Autodesk Inventor part; units mm, degrees
ref_plane "Work Plane1" through (0, 0, -15) normal (0, 0, 1) x (1, 0, 0)
ref_plane "YZ Plane" through (0, 0, 0) normal (1, 0, 0) x (0, 1, 0)
ref_plane "XZ Plane" through (0, 0, 0) normal (0, 1, 0) x (-1, 0, 0)
sketch "Sketch1" plane through (0, 0, 0) normal (0, 0, 1) x (1, 0, 0)
  line L0 (0, 0) -> (25, 0)
  line L1 (25, 0) -> (25, 40)
  line L2 (25, 40) -> (0, 40)
  line L3 (0, 40) -> (0, 0)
  dimension "d1" = 25
  dimension "d2" = 40
  dimension "d3" = 25
extrude "Extrusion1" add sketch "Sketch1" against normal blind 30
sketch "Sketch2" plane through (25, 0, 0) normal (1, 0, 0) x (0, 0, -1)
  line L0 (0, 0) -> (30, 0)
  circle A0 centre (15, 6.56) radius 2.46
extrude "Extrusion2" cut sketch "Sketch2" against normal blind 30
sketch "Sketch3" plane through (0, 0, 0) normal (-1, 0, 0) x (0, 0, 1)
  line L0 (0, 0) -> (-30, 0)
  line L1 (-25.05, 0) -> (-4.95, 0)
  line L2 (-4.95, 0) -> (-4.95, 33.12)
  line L3 (-4.95, 33.12) -> (-25.05, 33.12)
  line L4 (-25.05, 33.12) -> (-25.05, 0)
  dimension "d11" = 20.1
extrude "Extrusion3" cut sketch "Sketch3" against normal blind 20
sketch "Sketch4" plane through (0, 0, 0) normal (0, -1, 0) x (1, 0, 0)
  line L0 (20, -4.95) -> (20, -25.05)
  line L1 (20, -15) -> (25, -15)
  line L2 (25, 0) -> (25, -30)
  line L3 (20, -8.025) -> (25, -8.025)
  line L4 (25, -8.025) -> (25, -21.975)
  line L5 (25, -21.975) -> (20, -21.975)
  line L6 (20, -21.975) -> (20, -8.025)
  line L7 (20, -8.025) -> (25, -21.975) construction
  line L8 (25, -8.025) -> (20, -21.975) construction
  line L9 (25, -12.54) -> (25, -17.46)
  point P0 (0, 0)
  point P1 (22.5, -15)
  dimension "d14" = 13.95
extrude "Extrusion4" add sketch "Sketch4" along normal blind 15
sketch "Sketch5" plane through (20, 0, 0) normal (-1, 0, 0) x (0, 0, 1)
  circle A0 centre (-15, 6.56) radius 2.46
  circle A1 centre (-15, 6.56) radius 4.7025
  circle A2 centre (-15, 6.56) radius 2.46
  circle A3 centre (-15, 6.56) radius 2.46
  point P0 (0, 0)
  dimension "d17" = 9.405
extrude "Extrusion5" cut sketch "Sketch5" against normal blind 2.1
sketch "Sketch6" plane through (25, 0, 0) normal (1, 0, 0) x (0, 0, -1)
  circle A0 centre (15, 6.56) radius 4.7025
  line L0 (15, 6.56) -> (15, 23.56)
  circle A1 centre (15, 23.56) radius 2.46
  point P0 (0, 0)
  dimension "d20" = 17
  dimension "d21" = 4.92
extrude "Extrusion6" cut sketch "Sketch6" against normal blind 10 contours A1
sketch "Sketch7" plane through (20, 0, 0) normal (-1, 0, 0) x (0, 0, 1)
  circle A0 centre (-15, 23.56) radius 2.46
  circle A1 centre (-15, 23.56) radius 4.7025
  point P0 (0, 0)
  dimension "d24" = 9.405
extrude "Extrusion7" cut sketch "Sketch7" against normal blind 2.1
sketch "Sketch9" plane through (25, 0, 0) normal (1, 0, 0) x (0, 0, -1)
  circle A0 centre (15, 6.56) radius 2.46
  circle A1 centre (15, 6.56) radius 2.46
  circle A2 centre (15, 23.56) radius 2.46
  circle A3 centre (15, 23.56) radius 2.46
  line L0 (30, 40) -> (30, 0)
  line L1 (30, 0) -> (30, 40)
  line L2 (30, 40) -> (0, 40)
  line L3 (0, 40) -> (0, 0)
  line L4 (0, 0) -> (8.025, 0)
  line L5 (21.975, 0) -> (21.975, -15)
  line L6 (21.975, -15) -> (8.025, -15)
  line L7 (8.025, -15) -> (8.025, 0)
  line L8 (0, 0) -> (8.025, 0)
  line L9 (21.975, 0) -> (30, 0)
extrude "Extrusion8" add sketch "Sketch9" along normal blind 5
sketch "Sketch10" plane through (0, 40, 0) normal (0, 1, 0) x (1, 0, 0)
  line L0 (0, 30) -> (30, 30)
  line L1 (30, 0) -> (0, 0)
  line L2 (0, 30) -> (30, 30)
  line L3 (30, 30) -> (30, 0)
  line L4 (30, 0) -> (0, 0)
  line L5 (0, 0) -> (0, 30)
extrude "Extrusion9" add sketch "Sketch10" along normal blind 30
sketch "Sketch12" plane through (30, 0, 0) normal (1, 0, 0) x (0, 0, -1)
  circle A0 centre (15, 6.56) radius 2.46
  line L0 (15, 6.56) -> (15, 15.06)
  circle A1 centre (15, 15.06) radius 2.525
  point P0 (0, 0)
  dimension "d31" = 8.5
  dimension "d33" = 5.05
extrude "Extrusion10" cut sketch "Sketch12" against normal blind 30 contours A1
sketch "Sketch14" plane through (0, 0, 0) normal (0, 0, 1) x (1, 0, 0)
  line L0 (30, 70) -> (0, 70)
  line L1 (0, 70) -> (0, 85)
  line L2 (30, 100) -> (15, 115)
  line L3 (-12, 115) -> (15, 115)
  line L4 (30, 0) -> (30, 70)
  line L5 (30, 100) -> (30, 70)
  line L6 (-9.5, 113.5) -> (-12, 115)
  line L7 (-9.5, 101.5) -> (-12, 100)
  line L8 (-7, 107.5) -> (-9.5, 101.5)
  line L9 (-7, 107.5) -> (-9.5, 113.5)
  line L10 (0, 100) -> (0, 85)
  line L11 (0, 100) -> (-12, 100)
  point P0 (0, 0)
  dimension "d49" = 15
  dimension "d61" = 12
extrude "Extrusion12" add sketch "Sketch14" against normal blind 30
sketch "Sketch15" plane through (0, 0, -25.05) normal (-1, 0, 0) x (0, 0, 1)
  line L0 (0, 33.12) -> (20.1, 33.12)
  line L1 (20.1, 33.12) -> (20.1, 0)
  line L2 (0, 33.12) -> (20.1, 33.12)
  line L3 (20.1, 33.12) -> (20.1, 31.1)
  line L4 (20.1, 31.1) -> (0, 31.1)
  line L5 (0, 31.1) -> (0, 33.12)
  point P0 (25.05, 0)
  dimension "d57" = 2.02
extrude "Extrusion13" add sketch "Sketch15" against normal blind 20
sketch "Sketch19" plane through (0, 0, 0) normal (0, 0, 1) x (1, 0, 0)
  line L0 (0, 100) -> (0, 0)
  line L1 (0, 100) -> (-12, 100)
  line L2 (0, 100) -> (-12, 100)
  line L3 (-12, 100) -> (-9.5, 101.5)
  line L4 (-12, 100) -> (-9.5, 101.5)
  line L5 (-9.5, 101.5) -> (-7, 107.5)
  line L6 (-9.5, 101.5) -> (-7, 107.5)
  line L7 (-7, 107.5) -> (-9.5, 113.5)
  line L8 (-7, 107.5) -> (-9.5, 113.5)
  line L9 (-9.5, 113.5) -> (-12, 115)
  line L10 (-9.5, 113.5) -> (-12, 115)
  line L11 (-12, 115) -> (15, 115)
  line L12 (-12, 115) -> (15, 115)
  line L13 (15, 115) -> (30, 100)
  line L14 (15, 115) -> (30, 100)
  line L15 (30, 100) -> (30, 90)
  line L16 (30, 0) -> (30, 100)
  line L17 (30, 90) -> (0, 90)
  line L18 (0, 0) -> (0, 100)
  line L19 (0, 90) -> (0, 100)
  dimension "d62" = 10
  dimension "d63" = 30
extrude "Extrusion14" add sketch "Sketch19" along normal blind 30
ref_plane "Work Plane1" through (0, 0, -15) normal (0, 0, 1) x (1, 0, 0)
mirror "Mirror1" about plane through (0, 0, -15) normal (0, 0, 1) of "Extrusion14"
properties part number "rec_b_12mm_x_90mm"
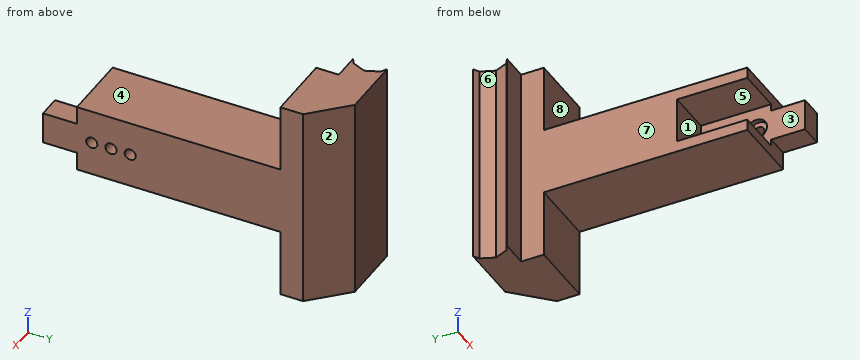
The model under review builds one solid part; all positions refer to its coordinate system, in mm. Face numbers are marked on the shaded views. A direction names the side the tool comes from. Round coordinates to 2 decimals unless told otherwise and drop trailing zeros. Loops run counter-clockwise (first coordinate to the right, second up) from the corner with the lowest first, then second, coordinate; pieces in that order, holes last. Notation, with made-up numbers: M -38.75,26 L 20.25,26 A29 ccw 20.25,53 Z; hole C 88.25,-35 d10. An arc over 180 degrees is marked long. Answer as a JSON object with one key per item and string values.
(1) To check wall thickness, follow line 1 along Z through (x, y) = (24.25, 6.56); line 2 along Y through (x, z) = (-9.5, -8); line 3 along Y through (x, z) = (26, -14). State the ranges of each line that lie inside material, in increasing order.
Resolved:
{"line 1": "-30 to -17.46, -12.54 to 0", "line 2": "100 to 101.5, 113.5 to 115", "line 3": "-15 to 4.31, 8.81 to 12.74, 17.38 to 21.31, 25.81 to 104"}
(2) Tool access review of the marked faces 5, 6, 7 and 8: name each direction out of +Z, -Z, +X, -X, +Y, -Y from which nothing blocks a thin tool from reaching the whole face with its end or side.
Resolved:
{"face 5": "-X, -Y", "face 6": "+Z, -Z, -X", "face 7": "+Z, -Z, -X, -Y", "face 8": "+Z, +X, -X, -Y"}
(3) Take a section at B-B on x = 7. Give the boundary of the cut face in (y, z).
Resolved:
{"outline": "M 0,-30 L 90,-30 L 90,-60 L 115,-60 L 115,30 L 90,30 L 90,0 L 0,0 L 0,-4.95 L 31.1,-4.95 L 31.1,-25.05 L 0,-25.05 Z"}
(4) Take a section at A-A on y = 6.56. Give the boundary of the cut face in (x, z), and give its area (3 significant figures).
Resolved:
{"outline": "M 0,-30 L 30,-30 L 30,-17.46 L 22.1,-17.46 L 22.1,-19.7 L 20,-19.7 L 20,-25.05 L 0,-25.05 Z; M 0,-4.95 L 20,-4.95 L 20,-10.3 L 22.1,-10.3 L 22.1,-12.54 L 30,-12.54 L 30,0 L 0,0 Z", "area": "439 mm²"}
(5) Take a section at D-D on x = 18.5. Give the boundary of the cut face in (y, z), and give its area (3 significant figures).
Resolved:
{"outline": "M 0,-30 L 90,-30 L 90,-60 L 111.5,-60 L 111.5,30 L 90,30 L 90,0 L 0,0 L 0,-4.95 L 31.1,-4.95 L 31.1,-25.05 L 0,-25.05 Z", "area": "4,010 mm²"}
(6) Clearance check with flat-ended pins moving along their axes: P1, Ø12, axis at y = 23.56, z = -15, coming from the +X side; P2, Ø6, axis at x = -5.5, z = -32, coming from the -Y side; P3, Ø9, axis at x = 8.5, z = -4.5, coming from the -Y side; P4, Ø5, axis at x = 27, y = -5, coming from the +Z side (3 decimals). State where each tip first meets the part, or that it passes through.
Resolved:
{"P1": "x = 30", "P2": "y = 100", "P3": "y = 0", "P4": "z = -8.025"}
(7) Draft analysis for pull direction Z (two halves, no side actions). For the marked faces 1, 2, 3 and 4, state which applies: released by +Z, released by -Z, zero draft, split by the parting line, or undercut.
Resolved:
{"face 1": "undercut", "face 2": "zero draft", "face 3": "undercut", "face 4": "released by +Z"}
(8) Take a section at C-C on z = -2. Give the boundary of the cut face in (x, y), and give its area (3 significant figures).
Resolved:
{"outline": "M -12,100 L 0,100 L 0,0 L 30,0 L 30,100 L 15,115 L -12,115 L -9.5,113.5 L -7,107.5 L -9.5,101.5 Z", "area": "3,470 mm²"}
